Design review of the part built by this model. Coordinates are the model's own, in mm. A direction names the side the tool comes from. Give positions to 0.01 mm unless a question says otherwise; leave off trailing zeros. Order: outer loops, then holes, each group sorted by start corner. A loop starts at its lowest first (then second) coordinate and runs counter-clockwise, first axis right, second up. Notation, with made-up numbers: (35, 13.25) -> (64, 13.25) arc R24 cw to (64, 47.25) -> close; hole circle Ø8 at (52.5, 83.25). An arc over 180 degrees is marked (long way). Answer in a Markdown table with one row per item. Add a question column.
```python
from build123d import *

# Parameters (mm, degrees)
SKETCH1_R           = 5.715
BOSS_EXTRUDE1_DEPTH = 6.35
SKETCH3_R           = 3.81
CUT_EXTRUDE1_DEPTH  = 6.35
BOSS_EXTRUDE3_DEPTH = 6.35
FILLET2_R           = 0.254
FILLET3_R           = 3.81
SKETCH4_W           = 6.35
SKETCH4_H           = 6.35
BOSS_EXTRUDE4_DEPTH = 6.35
SKETCH5_W           = 4.085425086
SKETCH5_H           = 2.54
CUT_EXTRUDE2_DEPTH  = 6.35
FILLET4_R           = 1.27


with BuildPart() as part:
    # Sketch1 → Boss-Extrude1 (new body)
    with BuildSketch(Plane(origin=(0, 0, 0), x_dir=(1, 0, 0), z_dir=(0, 1, 0))):
        with Locations(Location((0, 0, 0), (0, 0, 270))):
            Circle(SKETCH1_R)
    extrude(amount=BOSS_EXTRUDE1_DEPTH)

    # Sketch3 → Cut-Extrude1 (cut)
    with BuildSketch(Plane(origin=(0, 6.35, 0), x_dir=(1, 0, 0), z_dir=(0, 1, 0))):
        with Locations(Location((0, 0, 0), (0, 0, 270))):
            Circle(SKETCH3_R)
    extrude(amount=-CUT_EXTRUDE1_DEPTH, mode=Mode.SUBTRACT)

    # Sketch2 → Boss-Extrude3 (add)
    with BuildSketch(Plane(origin=(0, 6.35, 0), x_dir=(1, 0, 0), z_dir=(0, 1, 0))):
        Polygon((5.08, 2.618172072), (8.876921418, -8.162750326), (2.764587199, -5.001827928), align=None)
    extrude(amount=-BOSS_EXTRUDE3_DEPTH)

    # Fillet2
    fillet2_edges = [part.edges().sort_by_distance(p)[0] for p in [
        (8.876921418, 3.175, 8.162750326),
    ]]
    fillet(fillet2_edges, radius=FILLET2_R)

    # Fillet3
    fillet3_edges = [part.edges().sort_by_distance(p)[0] for p in [
        (2.764587199, 3.175, 5.001827928),
    ]]
    fillet(fillet3_edges, radius=FILLET3_R)

    # Sketch4 → Boss-Extrude4 (add)
    with BuildSketch(Plane(origin=(0, 6.35, 0), x_dir=(1, 0, 0), z_dir=(0, 1, 0))):
        with Locations((0, 7.926904881)):
            Rectangle(SKETCH4_W, SKETCH4_H)
    extrude(amount=-BOSS_EXTRUDE4_DEPTH)

    # Sketch5 → Cut-Extrude2 (cut)
    with BuildSketch(Plane(origin=(0, 6.35, 0), x_dir=(1, 0, 0), z_dir=(0, 1, 0))):
        with Locations((-1.132287457, 7.291904881)):
            Rectangle(SKETCH5_W, SKETCH5_H)
    extrude(amount=-CUT_EXTRUDE2_DEPTH, mode=Mode.SUBTRACT)

    # Fillet4
    fillet4_edges = [part.edges().sort_by_distance(p)[0] for p in [
        (3.175, 3.175, -4.751904881),
        (-3.175, 3.175, -6.021904881),
        (0.910425086, 3.175, -6.021904881),
        (0.910425086, 3.175, -8.561904881),
        (-3.175, 3.175, -8.561904881),
        (-3.175, 3.175, -11.101904881),
        (3.175, 3.175, -11.101904881),
    ]]
    fillet(fillet4_edges, radius=FILLET4_R - 0.0001)  # a hair under: the kernel refuses the full size


solid = part.part
```
1) Clearance check with flat-ended pins moving along their axes: P1, Ø1, axis at y = 2.5, z = -7, coming from the -X side; P2, Ø1.7, axis at x = -1, y = 3, coming from the +Z side; P3, Ø2, axis at y = 4.5, z = -8, coming from the +X side (3 decimals). State where each tip first meets the part, or that it passes through.
2) Add section A-A, the plane z = 0. Write out the cut boundary in (x, y) (3 decimals), and give its area (3 significant figures).
3) Machinability: for faces 5 (the face through (-1, 3, -6.022)), 6 (the face through (3.293, 3.131, -4.854)), which of the approach directions +Z, -Z, +X, -X, +Y, -Y give a long, thin tool a straight path to every point of the face, cutting with its end or side? Answer none if there is none.
4) Add section D-D, the plane z = 2.5. Write out the cut boundary in (x, y).
5) Add section B-B, the plane x = 0. Write out the cut boundary in (y, z) (3 decimals), and give its area (3 significant figures).
6) Mouldability with a two-part tool opening along Z and no side actions: class faces 1 (the face through (-2.79, 3.13, -8.92)), 2 (the face through (-1, 3, -8.562)), 3 (the face through (2.96, 3.13, 5.39)), 4 (the face through (3.175, 3, -8)) as +Z half, -Z half, draft (parallel to the pull), parting line (faces both ways), or undercut.
7) For L1, parallel to Z at x = 0.25, y = 3.75; L2, parallel to X at y = 3.25, z = 0 (3 decimals); L3, parallel to Z at x = 2.75, y = 2, list the stretches that pass through material, from the lowest coordinate up.
Verdict:
| question | item | result |
|---|---|---|
| 1 | P1 | stops at x = 0.63 |
| 1 | P2 | stops at z = 5.71 |
| 1 | P3 | stops at x = 3.175 |
| 2 | outline | (-5.715, 0) -> (-3.81, 0) -> (-3.81, 6.35) -> (-5.715, 6.35) -> close; (3.81, 0) -> (6.002, 0) -> (6.002, 6.35) -> (3.81, 6.35) -> close |
| 2 | area | 26.0 mm2 |
| 3 | face 5 | -X, +Y, -Y |
| 3 | face 6 | -Z, +X, +Y, -Y |
| 4 | outline | (-5.14, 0) -> (-2.88, 0) -> (-2.88, 6.35) -> (-5.14, 6.35) -> close; (2.88, 0) -> (6.88, 0) -> (6.88, 6.35) -> (2.88, 6.35) -> close |
| 5 | outline | (0, -11.102) -> (6.35, -11.102) -> (6.35, -8.51) -> (0, -8.51) -> close; (0, -6.074) -> (6.35, -6.074) -> (6.35, -3.81) -> (0, -3.81) -> close; (0, 3.81) -> (6.35, 3.81) -> (6.35, 5.715) -> (0, 5.715) -> close |
| 5 | area | 42.9 mm2 |
| 6 | face 1 | undercut |
| 6 | face 2 | undercut |
| 6 | face 3 | +Z half |
| 6 | face 4 | draft |
| 7 | L1 | z = -11.1 to -8.41, -6.18 to -3.8, 3.8 to 5.71 |
| 7 | L2 | x = -5.715 to -3.81, 3.81 to 6.002 |
| 7 | L3 | z = -10.78 to -2.64, 2.64 to 5.37 |
